from build123d import *

# Parameters (mm, degrees)
BOSS_EXTRUDE1_DEPTH     = 15
CUT_EXTRUDE1_DEPTH      = 77.635500912
CUT_EXTRUDE1_DEPTH_BACK = 77.635500912
SKETCH3_R               = 2.5


with BuildPart() as part:
    # Sketch1 → Boss-Extrude1 (new, symmetric)
    with BuildSketch(Plane.XY):
        Polygon((-15, -8), (-15, 32), (15, 32), (15, -8), (15.5, -8), (16, 0), (16, 68), (-16, 68), (-16, 0), (-15.5, -8), align=None)
    extrude(amount=BOSS_EXTRUDE1_DEPTH, both=True)

    # Sketch3 → Cut-Extrude1 (cut, two sides: drawn at the far end of the back side and taken through both)
    with BuildSketch(Plane.ZY.offset(16).offset(-CUT_EXTRUDE1_DEPTH_BACK)):
        Circle(SKETCH3_R)
        with BuildLine():
            Line((-10, 0), (-10, 50))
            Line((-10, 50), (-16.325920345, 54.897216738))
            Line((-16.325920345, 54.897216738), (-25.192820329, 54.897216738))
            Line((-25.192820329, 54.897216738), (-25.192820329, -12.983802327))
            Line((-25.192820329, -12.983802327), (26.325920345, -12.983802327))
            Line((26.325920345, -12.983802327), (26.325920345, 54.897216738))
            Line((26.325920345, 54.897216738), (16.325920345, 54.897216738))
            Line((16.325920345, 54.897216738), (10, 50))
            Line((10, 50), (10, 0))
            ThreePointArc((10, 0), (0, -7.874716557), (-10, 0))
        make_face()
    extrude(amount=CUT_EXTRUDE1_DEPTH + CUT_EXTRUDE1_DEPTH_BACK, mode=Mode.SUBTRACT)


solid = part.part
Input: part model. Units: mm. Frame: model coordinates. A direction names the side the tool comes from. Coordinates: 2 decimals unless noted, no trailing zeros. Loops run counter-clockwise (first coordinate to the right, second up) from the corner with the lowest first, then second, coordinate; pieces in that order, holes last.
Q1. Material intervals for line 1 (Z direction, x = -15.5, y = 0); line 2 (X direction, y = 5, z = 8); line 3 (Z direction, x = 3, y = 39), sorted ascending.
Q2. Set-up query: faces 4 (the face through (1, 38, -10)), 5 (the face through (-16, 34, 0)), 6 (the face through (-2, 38, 10)), 7 (the face through (0, 32, 0)). Return all of +Z, -Z, +X, -X, +Y, -Y with unobstructed straight access to the full face (end or side cutting, diameter ignored); none if empty.
Q3. Cut plane C-C (z = 0). Output: boundary loops of the cut face in (x, y), then the cut area to 3 significant figures.
Q4. Draft query along Z for faces 1 (the face through (-15.271, -7.873, 0.192)), 2 (the face through (-15.49, 2.11, 1.34)), 3 (the face through (15.75, -3.99, 0.14)). Return one class per face: +Z half, -Z half, draft (parallel to the pull), parting line (faces both ways), or undercut.
Q5. Cut plane A-A (y = 28). Output: boundary loops of the cut face in (x, z).
Q6. Cut plane D-D (z = 5.5). Output: boundary loops of the cut face in (x, y), then the cut area to 3 significant figures.
Q7. Cut plane B-B (x = 0.5). Output: boundary loops of the cut face in (y, z), then the cut area to 3 significant figures.
Q8. Contact query for flat-ended pins moving along their axis: pin 1 (3 mm diameter, centred on x = 10, z = 0.5, fed in from -Y); pin 2 (4 mm diameter, centred on x = 11.5, y = 37, fed in from +Z). Output: stop coordinate, or through.
Working result:
1. line 1: z = -10 to -2.5, 2.5 to 10
1. line 2: x = -16 to -15, 15 to 16
1. line 3: z = -10 to 10
2. face 4: -Z, +X, -X, -Y
2. face 5: +Z, -Z, -X, +Y, -Y
2. face 6: +Z, +X, -X, -Y
2. face 7: +Z, -Z, -Y
3. outline: (-16, 2.5) - (-15, 2.5) - (-15, 32) - (15, 32) - (15, 2.5) - (16, 2.5) - (16, 68) - (-16, 68) - close; (-15.84, -2.5) - (-15.51, -7.87) - (-15, -7.87) - (-15, -2.5) - close; (15, -7.87) - (15.51, -7.87) - (15.84, -2.5) - (15, -2.5) - close
3. area: 1,220 mm2
4. face 1: parting line
4. face 2: undercut
4. face 3: draft
5. outline: (-16, -10) - (-15, -10) - (-15, 10) - (-16, 10) - close; (15, -10) - (16, -10) - (16, 10) - (15, 10) - close
6. outline: (-16, 0) - (-15.61, -6.28) - (-15, -6.28) - (-15, 32) - (15, 32) - (15, -6.28) - (15.61, -6.28) - (16, 0) - (16, 68) - (-16, 68) - close
6. area: 1,230 mm2
7. outline: (32, -10) - (50, -10) - (53.87, -15) - (68, -15) - (68, 15) - (53.87, 15) - (50, 10) - (32, 10) - close
7. area: 881 mm2
8. pin 1: stops at y = 32
8. pin 2: stops at z = 10
